Study the drawing (mm; zero at the part's minimum x, y, z) and answer. A direction names the side the tool comes from. Coordinates: 2 decimals unless noted, no trailing zeros. Loops run counter-clockwise (first coordinate to the right, second up) from the corner with the lowest first, then second, coordinate; pieces in that order, holes last. Notation, with made-up numbers: (11, -2) -> (43, -2) arc R30 ccw to (43, 34) -> close; hole circle Ø10 at (24.25, 83.25). An arc over 180 degrees is marked (long way). Answer in a Markdown table with one row per item.
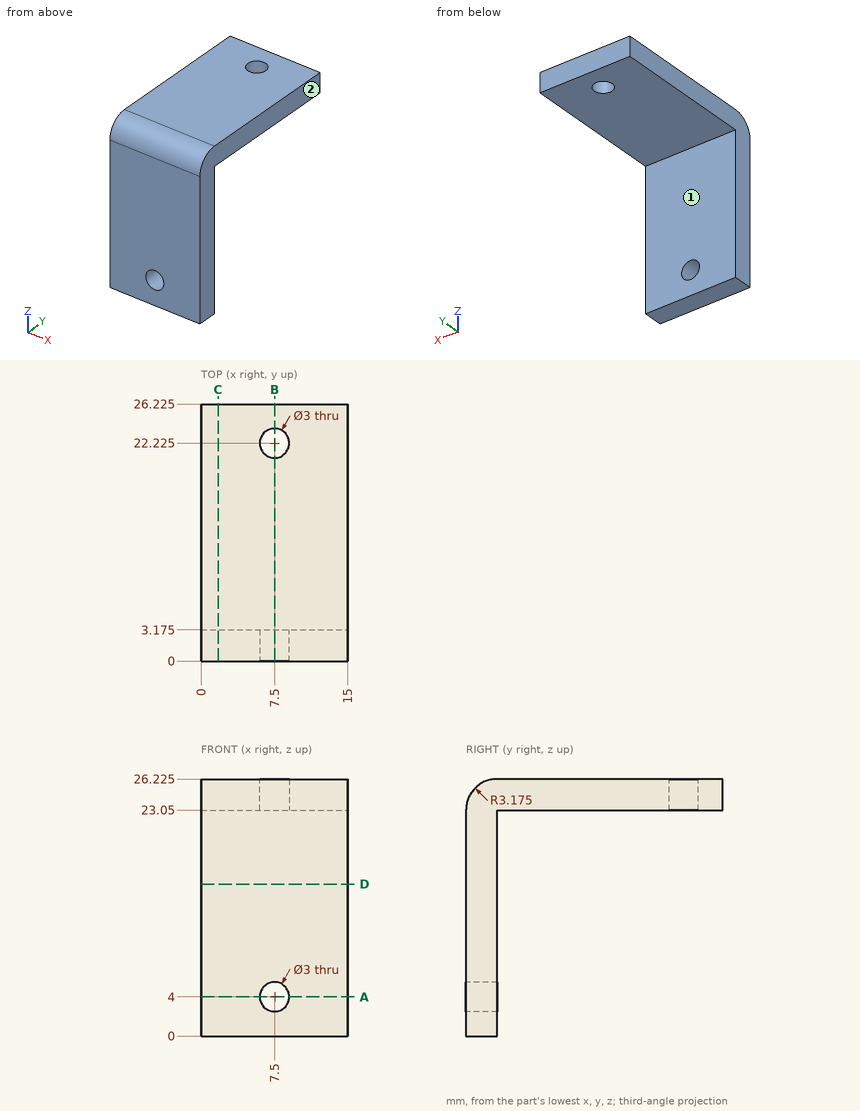
1. Find the intervals of material crossed by probe 1 along Z at (x, y) = (8, 24.5) (3 decimals); probe 2 along Y at (x, z) = (9, 18) (3 decimals); probe 3 along Y at (x, z) = (6.25, 23.5) (3 decimals), in increasing order.
A:
| item | result |
|---|---|
| probe 1 | z = 23.05 to 26.225 |
| probe 2 | y = 0 to 3.175 |
| probe 3 | y = 0.032 to 21.396, 23.054 to 26.225 |
2. A cutting plane is placed at C-C on x = 1.75. Give the vertices of the cut face in (y, z) (3 decimals).
A:
| item | result |
|---|---|
| outline | (0, 0) -> (3.175, 0) -> (3.175, 23.05) -> (26.225, 23.05) -> (26.225, 26.225) -> (3.175, 26.225) arc R3.175 ccw to (0, 23.05) -> close |
3. Given pin 1 Ø1 at (x, z) = (11, 12) entering from +Y (3 decimals); pin 2 Ø2 at (x, y) = (11.5, 18.5) entering from -Z; pin 3 Ø10 at (y, z) = (6.5, 12.5) entering from +X, each flat-ended and moving along its own axis, determine where each tip first touches the part or whether it passes through.
A:
| item | result |
|---|---|
| pin 1 | stops at y = 3.175 |
| pin 2 | stops at z = 23.05 |
| pin 3 | stops at x = 15 |
4. A cutting plane is placed at B-B on x = 7.5. Give the vertices of the cut face in (y, z) (3 decimals).
A:
| item | result |
|---|---|
| outline | (0, 0) -> (3.175, 0) -> (3.175, 2.5) -> (0, 2.5) -> close; (0, 5.5) -> (3.175, 5.5) -> (3.175, 23.05) -> (20.725, 23.05) -> (20.725, 26.225) -> (3.175, 26.225) arc R3.175 ccw to (0, 23.05) -> close; (23.725, 23.05) -> (26.225, 23.05) -> (26.225, 26.225) -> (23.725, 26.225) -> close |
5. A cutting plane is placed at D-D on z = 15.5. Give the vertices of the cut face in (x, y) (3 decimals).
A:
| item | result |
|---|---|
| outline | (0, 0) -> (15, 0) -> (15, 3.175) -> (0, 3.175) -> close |
6. A tool of negligible diameter and unlimited length cuts with its end or side. For the marked faces 1 and 2, from which of +Z, -Z, +X, -X, +Y, -Y can it reach the whole face along a straight path? Write none if from no direction.
A:
| item | result |
|---|---|
| face 1 | -Z, +X, -X, +Y |
| face 2 | +Z, -Z, +X, +Y, -Y |
7. A cutting plane is placed at A-A on z = 4. Give the vertices of the cut face in (x, y) (3 decimals), and give its area (3 significant figures).
A:
| item | result |
|---|---|
| outline | (0, 0) -> (6, 0) -> (6, 3.175) -> (0, 3.175) -> close; (9, 0) -> (15, 0) -> (15, 3.175) -> (9, 3.175) -> close |
| area | 38.1 mm2 |
